Geometry: final body of the model. Coordinates: model frame, mm. Face numbers are marked on the shaded views. A direction names the side the tool comes from. Round coordinates to 2 decimals unless told otherwise and drop trailing zeros. Loops run counter-clockwise (first coordinate to the right, second up) from the corner with the lowest first, then second, coordinate; pieces in that order, holes last. Notation, with made-up numbers: (60.5, 1.25) -> (113.5, 1.25) arc R32 ccw to (113.5, 28.25) -> close; hole circle Ø7 at (73, 22). An arc over 180 degrees is marked (long way). Answer in a Markdown table with one row per item.
```python
from build123d import *

# Parameters (mm, degrees)
F0_W     = 70.067666
F0_H     = 70.067667
F2_DEPTH = 15
F1_W     = 5.398806
F1_H     = 5.399308
F1_H_2   = 5.399307
F3_DEPTH = 25


with BuildPart() as f2:
    # F0 (on Top) → F2 (new body)
    with BuildSketch(Plane.XY):
        with Locations((0.265833, -0.609237)):
            Rectangle(F0_W, F0_H)
    extrude(amount=F2_DEPTH)

    # F1 (on Top) → F3 (join)
    with BuildSketch(Plane.XY):
        Polygon((-14.17026, 16.568485), (-19.4919, 16.568485), (-19.4919, -24.765937), (-14.17026, -24.765937), (-14.17026, -19.366629), align=None)
        with Locations((-11.470857, -22.066283)):
            Rectangle(F1_W, F1_H)
        Polygon((-10.363362, 24.496303), (-19.585205, 24.496303), (-24.996936, 24.496303), (-24.996936, 27.575392), (-32.27913, 21.791303), (-24.996936, 16.007215), (-24.996936, 19.086303), (-19.585205, 19.086303), (-13.312519, 19.086303), (9.406068, -24.765937), (18.790985, -24.765937), (24.202717, -24.765937), (24.202717, -27.845025), (31.48491, -22.060937), (24.202717, -16.276848), (24.202717, -19.355937), (18.790985, -19.355937), (12.355225, -19.355937), align=None)
        Polygon((13.37604, -16.838118), (18.69768, -16.838118), (18.69768, 24.496303), (13.37604, 24.496303), (13.37604, 19.096996), align=None)
        with Locations((10.676637, 21.79665)):
            Rectangle(F1_W, F1_H_2)
    extrude(amount=F3_DEPTH)


solid = f2.part
```
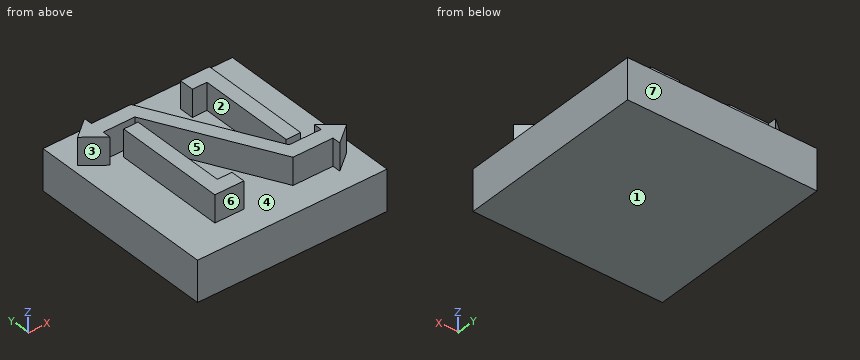
Item 1: Cut plane C-C (y = -23.5). Output: boundary loops of the cut face in (x, z).
Answer:
| item | result |
|---|---|
| outline | (-34.77, 0) -> (35.3, 0) -> (35.3, 15) -> (29.67, 15) -> (29.67, 25) -> (8.75, 25) -> (8.75, 15) -> (-8.77, 15) -> (-8.77, 25) -> (-19.49, 25) -> (-19.49, 15) -> (-34.77, 15) -> close |
Item 2: Line query: probe 1 along X at (y, z) = (-2.5, 19.5); probe 2 along Y at (x, z) = (-14.5, 21.5); probe 3 along Z at (x, y) = (32.5, 31.5). Output: solid intervals per line, ascending. Write a range as [from, to].
Answer:
| item | result |
|---|---|
| probe 1 | x = [-19.49, -14.17], [-2.13, 3.62], [13.38, 18.7] |
| probe 2 | y = [-24.77, 16.57], [19.09, 24.5] |
| probe 3 | z = [0, 15] |
Item 3: Cut plane D-D (y = 5). Output: boundary loops of the cut face in (x, z).
Answer:
| item | result |
|---|---|
| outline | (-34.77, 0) -> (35.3, 0) -> (35.3, 15) -> (18.7, 15) -> (18.7, 25) -> (13.38, 25) -> (13.38, 15) -> (-0.26, 15) -> (-0.26, 25) -> (-6.01, 25) -> (-6.01, 15) -> (-14.17, 15) -> (-14.17, 25) -> (-19.49, 25) -> (-19.49, 15) -> (-34.77, 15) -> close |
Item 4: Pin query (flat end, axial travel): pin 1 Ø2.5 at (x, z) = (11.5, 18.5) entering from +Y; pin 2 Ø6 at (y, z) = (-22, 19.5) entering from +X; pin 3 Ø12 at (x, z) = (23.5, 22.5) entering from -Y (3 decimals). Return the tip coordinate at first contact, or that it passes through.
Answer:
| item | result |
|---|---|
| pin 1 | stops at y = 24.5 |
| pin 2 | stops at x = 31.48 |
| pin 3 | stops at y = -27.845 |
Item 5: Draft query along X for the marked faces 1, 2, 3 and 4. Return one class per face: pulls with the +X half, pulls with the -X half, needs draft (parallel to the pull), parting line crosses it, or undercut.
Answer:
| item | result |
|---|---|
| face 1 | needs draft |
| face 2 | undercut |
| face 3 | pulls with the -X half |
| face 4 | undercut |
Item 6: Cut plane A-A (z = 20.5). Output: boundary loops of the cut face in (x, y), then the cut area to 3 significant figures.
Answer:
| item | result |
|---|---|
| outline | (-32.28, 21.79) -> (-25, 16.01) -> (-25, 19.09) -> (-13.31, 19.09) -> (9.41, -24.77) -> (24.2, -24.77) -> (24.2, -27.85) -> (31.48, -22.06) -> (24.2, -16.28) -> (24.2, -19.36) -> (12.36, -19.36) -> (-10.36, 24.5) -> (-25, 24.5) -> (-25, 27.58) -> close; (-19.49, -24.77) -> (-8.77, -24.77) -> (-8.77, -19.37) -> (-14.17, -19.37) -> (-14.17, 16.57) -> (-19.49, 16.57) -> close; (7.98, 19.1) -> (13.38, 19.1) -> (13.38, -16.84) -> (18.7, -16.84) -> (18.7, 24.5) -> (7.98, 24.5) -> close |
| area | 978 mm² |
Item 7: Cut plane B-B (x = 22.5). Output: boundary loops of the cut face in (y, z).
Answer:
| item | result |
|---|---|
| outline | (-35.64, 0) -> (34.42, 0) -> (34.42, 15) -> (-19.36, 15) -> (-19.36, 25) -> (-24.77, 25) -> (-24.77, 15) -> (-35.64, 15) -> close |
Item 8: Reachability of the marked faces 5, 6 and 7 from +Z, -Z, +X, -X, +Y, -Y: full face, straight path, thin tool, end or side. Return the list, or none.
Answer:
| item | result |
|---|---|
| face 5 | +Z |
| face 6 | +Z, -X, -Y |
| face 7 | +Z, -Z, +X, -X, +Y |
